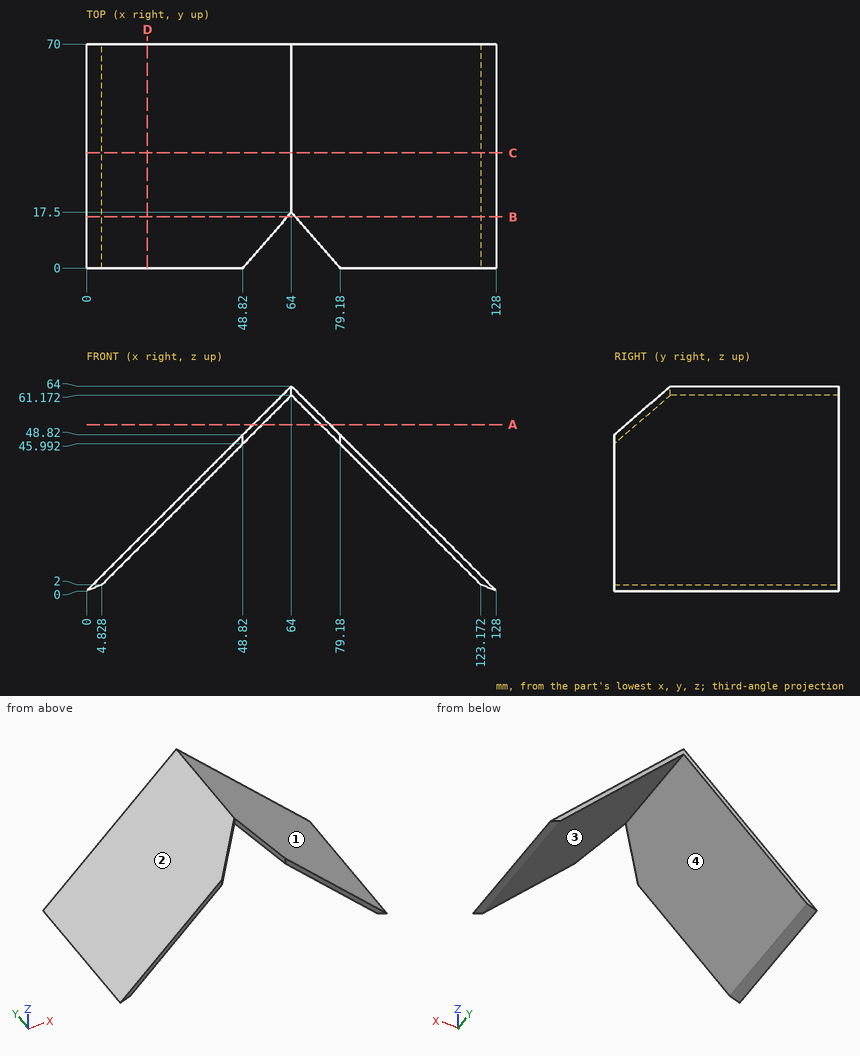
For this review, use the dimensioned drawing (mm, ordinates from the lowest corner) and the shaded views. Give positions to 0.01 mm unless a question says otherwise; leave off trailing zeros. Order: outer loops, then holes, each group sorted by start corner. A loop starts at its lowest first (then second) coordinate and runs counter-clockwise, first axis right, second up.
1. Mouldability with a two-part tool opening along X and no side actions: class the marked faces 1, 2, 3 and 4 as +X half, -X half, draft (parallel to the pull), parting line (faces both ways), or undercut.
Solution:
face 1: +X half
face 2: -X half
face 3: undercut
face 4: undercut
2. Add section C-C, the plane y = 36. State the section outline as (x, z) points.
Solution:
outline: (0, 0) - (4.83, 2) - (64, 61.17) - (123.17, 2) - (128, 0) - (64, 64) - close
3. To check wall thickness, follow L1, parallel to X at y = 56, z = 46; L2, parallel to X at y = 63, z = 39; L3, parallel to Z at x = 77.5, y = 9. State the ranges of each line that lie inside material, in increasing order.
Solution:
L1: x = 46 to 48.83, 79.17 to 82
L2: x = 39 to 41.83, 86.17 to 89
L3: z = 47.67 to 50.5
4. Add section B-B, the plane y = 16. State the section outline as (x, z) points.
Solution:
outline: (0, 0) - (4.83, 2) - (62.7, 59.87) - (62.7, 62.7) - close; (65.3, 59.87) - (123.17, 2) - (128, 0) - (65.3, 62.7) - close
5. Add section A-A, the plane z = 52. State the section outline as (x, y) points, then the cut area to 3 significant figures.
Solution:
outline: (52, 3.67) - (54.83, 6.93) - (54.83, 70) - (52, 70) - close; (73.17, 6.93) - (76, 3.67) - (76, 70) - (73.17, 70) - close
area: 366 mm2
6. For pin 1 Ø6 at (x, z) = (51, 43.5) entering from +Y; pin 2 Ø12 at (x, y) = (21, 50) entering from -Z; pin 3 Ø8 at (y, z) = (10.5, 31) entering from -X; pin 4 Ø6 at (x, y) = (30, 50.5) entering from +Z, all flat-tipped, find the tip position at first contact; note any pin that passes through.
Solution:
pin 1: passes through
pin 2: stops at z = 12.17
pin 3: stops at x = 27
pin 4: stops at z = 33
7. Add section D-D, the plane x = 19. State the section outline as (y, z) points, then the cut area to 3 significant figures.
Solution:
outline: (0, 16.17) - (70, 16.17) - (70, 19) - (0, 19) - close
area: 198 mm2
